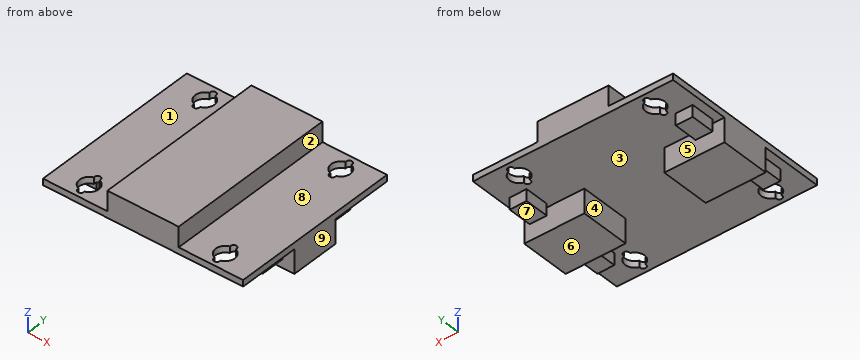
Autodesk Inventor part; units mm, degrees
ref_plane "YZ Plane" through (0, 0, 0) normal (1, 0, 0) x (0, 1, 0)
ref_plane "XZ Plane" through (0, 0, 0) normal (0, 1, 0) x (-1, 0, 0)
ref_plane "XY Plane" through (0, 0, 0) normal (0, 0, 1) x (1, 0, 0)
sketch "スケッチ1" plane through (0, 0, 0) normal (0, 0, 1) x (1, 0, 0)
  line L0 (-25, -21.59) -> (25, -21.59)
  line L1 (25, -21.59) -> (25, 21.59)
  line L2 (25, 21.59) -> (-25, 21.59)
  line L3 (-25, 21.59) -> (-25, -21.59)
  line L4 (-25, -21.59) -> (25, 21.59) construction
  line L5 (25, -21.59) -> (-25, 21.59) construction
  line L6 (-17, -17.34) -> (17, -17.34) construction
  line L7 (17, -17.34) -> (17, 17.34) construction
  line L8 (17, 17.34) -> (-17, 17.34) construction
  line L9 (-17, 17.34) -> (-17, -17.34) construction
  line L10 (-17, -17.34) -> (17, 17.34) construction
  line L11 (17, -17.34) -> (-17, 17.34) construction
  line L12 (-25, 6.2) -> (-10, 6.2)
  line L13 (-10, 6.2) -> (-10, -6.2)
  line L14 (-10, -6.2) -> (-25, -6.2)
  line L15 (-25, 0) -> (25, 0) construction
  line L16 (0, -21.59) -> (0, 21.59) construction
  line L17 (25, 6.2) -> (10, 6.2)
  line L18 (10, 6.2) -> (10, -6.2)
  line L19 (10, -6.2) -> (25, -6.2)
  line L20 (-8.89, -21.59) -> (8.89, -21.59)
  line L21 (8.89, -21.59) -> (8.89, 21.59)
  line L22 (8.89, 21.59) -> (-8.89, 21.59)
  line L23 (-8.89, 21.59) -> (-8.89, -21.59)
  line L24 (-8.89, -21.59) -> (8.89, 21.59) construction
  line L25 (8.89, -21.59) -> (-8.89, 21.59) construction
  circle A0 centre (17, 17.34) radius 2.4
  arc A1 (16.2801, 15.0505) -> (17.7199, 15.0505) centre (17, 14.84) ccw
  arc A2 (17.7199, 19.6295) -> (16.2801, 19.6295) centre (17, 19.84) ccw
  circle A3 centre (-17, 17.34) radius 2.4
  arc A4 (-16.2801, 19.6295) -> (-17.7199, 19.6295) centre (-17, 19.84) ccw
  arc A5 (-17.7199, 15.0505) -> (-16.2801, 15.0505) centre (-17, 14.84) ccw
  circle A6 centre (17, -17.34) radius 2.4
  arc A7 (16.2801, -19.6295) -> (17.7199, -19.6295) centre (17, -19.84) ccw
  arc A8 (17.7199, -15.0505) -> (16.2801, -15.0505) centre (17, -14.84) ccw
  circle A9 centre (-17, -17.34) radius 2.4
  arc A10 (-16.2801, -15.0505) -> (-17.7199, -15.0505) centre (-17, -14.84) ccw
  arc A11 (-17.7199, -19.6295) -> (-16.2801, -19.6295) centre (-17, -19.84) ccw
  line L26 (-22.86, -13.16) -> (-18.61, -13.16)
  line L27 (-18.61, -13.16) -> (-18.61, -7.16)
  line L28 (-18.61, -7.16) -> (-22.86, -7.16)
  line L29 (-22.86, -7.16) -> (-22.86, -13.16)
  line L30 (-22.86, -13.16) -> (-18.61, -7.16) construction
  line L31 (-18.61, -13.16) -> (-22.86, -7.16) construction
  line L32 (-22.86, 13.16) -> (-18.61, 13.16)
  line L33 (-18.61, 13.16) -> (-18.61, 7.16)
  line L34 (-18.61, 7.16) -> (-22.86, 7.16)
  line L35 (-22.86, 7.16) -> (-22.86, 13.16)
  line L36 (22.86, -13.16) -> (18.61, -13.16)
  line L37 (18.61, -13.16) -> (18.61, -7.16)
  line L38 (18.61, -7.16) -> (22.86, -7.16)
  line L39 (22.86, -7.16) -> (22.86, -13.16)
  line L40 (18.61, 13.16) -> (18.61, 7.16)
  line L41 (22.86, 13.16) -> (18.61, 13.16)
  line L42 (22.86, 7.16) -> (22.86, 13.16)
  line L43 (18.61, 7.16) -> (22.86, 7.16)
  point P0 (0, 0)
  point P1 (-10, 0)
  point P2 (25, 6.2)
  point P3 (25, -6.2)
  point P4 (0, 0)
  point P5 (0, 0)
  point P6 (0, 0)
  point P7 (17, 20.59)
  point P8 (17, 14.09)
  point P9 (-20.735, -10.16)
  point P10 (-22.86, -10.16)
  dimension "d0" = 50
  dimension "d1" = 43.18
  dimension "d2" = 34
  dimension "d3" = 34.68
  dimension "d8" = 15
  dimension "d9" = 12.4
  dimension "d17" = 17.78
  dimension "d18" = 43.18
  dimension "d25" = 16
  dimension "d26" = 4.8
  dimension "d27" = 6.5
  dimension "d28" = 1.5
  dimension "d29" = 1
  dimension "d30" = 8.5
  dimension "d31" = 16
  dimension "d32" = 4.25
  dimension "d33" = 6
  dimension "d34" = 10.16
  dimension "d35" = 22.86
extrude "押し出し1" add sketch "スケッチ1" along normal blind 1.6 contours L3 L14 L13 L12 L2 L23 L0 | L23 L2 L21 L0 | L3 L12 L13 L14 | L21 L2 L1 L17 L18 L19 L0 | L19 L18 L17 L1 | L29 L28 L27 L26 | L32 L33 L34 L35 | L36 L37 L38 L39 | L41 L42 L43 L40
extrude "押し出し2" add sketch "スケッチ1" against normal blind 6 contours L3 L12 L13 L14 | L19 L18 L17 L1
extrude "押し出し3" add sketch "スケッチ1" along normal blind 6.6 contours L23 L2 L21 L0
extrude "Extrusion4" add sketch "スケッチ1" against normal blind 2.9 contours L29 L28 L27 L26 | L32 L33 L34 L35 | L36 L37 L38 L39 | L41 L42 L43 L40
properties part number "SUSTAINA-STRAINGAUGE-SENSING-BOARD" material "Acetal Resin, Black"
Here's how the part is built. I have some questions about the finished solid (model axes, mm). Face numbers are marked on the shaded views. A direction names the side the tool comes from. Give positions to 0.01 mm unless a question says otherwise; leave off trailing zeros. Write each loop counter-clockwise with the first axis right and the second up, starting at its lowest first coordinate (ties: lowest second). Pieces come first, ordered by that corner, then holes.
(1) Imagine slicing it at C-C, the plane y = 9. Write out the boundary of the cut face in (x, z), and give its area (3 significant figures).
Output values:
outline: (-25, 0) - (-22.86, 0) - (-22.86, -2.9) - (-18.61, -2.9) - (-18.61, 0) - (18.61, 0) - (18.61, -2.9) - (22.86, -2.9) - (22.86, 0) - (25, 0) - (25, 1.6) - (8.89, 1.6) - (8.89, 6.6) - (-8.89, 6.6) - (-8.89, 1.6) - (-25, 1.6) - close
area: 194 mm2
(2) Thinking about a two-plate mould opening in X: for the marked faces 1, 2, 3 and 4, which applies, pulls with the +X half, pulls with the -X half, needs draft (parallel to the pull), parting line crosses it, or undercut?
Output values:
face 1: needs draft
face 2: pulls with the +X half
face 3: undercut
face 4: undercut
(3) If I drill on L1, parallel to X at y = 19.84, z = 1.1; L2, parallel to Y at x = -21.5, z = -0.5; L3, parallel to X at y = 18.5, z = 0.5, over which ranges is the centre line in solid material (lowest first)?
Output values:
L1: x = -25 to -17.75, -16.25 to 16.25, 17.75 to 25
L2: y = -13.16 to -7.16, -6.2 to 6.2, 7.16 to 13.16
L3: x = -25 to -19.1, -14.9 to 14.9, 19.1 to 25
(4) Will these pins go through, and if not, where does the flat tip stop? pin 1 (1.7 mm diameter, centred on x = -17, y = -14.84, fed in from +Z); pin 2 (2 mm diameter, centred on x = 17, y = 14.84, fed in from -Z); pin 3 (0.9 mm diameter, centred on x = 17, y = -19.84, fed in from -Z); pin 4 (1.4 mm diameter, centred on x = 21, z = -1, fed in from -Y).
Output values:
pin 1: stops at z = 1.6
pin 2: stops at z = 0
pin 3: passes through
pin 4: stops at y = -13.16
(5) On a 3-axis mill with a long thin cutter (end or side, diameter ignored), from which of +Z, -Z, +X, -X, +Y, -Y can I reach the whole of each face in a straight line? I mean the marked faces 5, 6, 7, 8 and 9. Say none if no direction works.
Output values:
face 5: -Z, +X, -X
face 6: -Z, +X, -X, +Y, -Y
face 7: -Z, +X, -X, +Y
face 8: +Z, +X, +Y, -Y
face 9: +Z, -Z, +X, +Y, -Y
(6) Imagine slicing it at B-B, the plane x = -17. Write out the boundary of the cut face in (y, z).
Output values:
outline: (-21.59, 0) - (-20.59, 0) - (-20.59, 1.6) - (-21.59, 1.6) - close; (-14.09, 0) - (-6.2, 0) - (-6.2, -6) - (6.2, -6) - (6.2, 0) - (14.09, 0) - (14.09, 1.6) - (-14.09, 1.6) - close; (20.59, 0) - (21.59, 0) - (21.59, 1.6) - (20.59, 1.6) - close
(7) Imagine slicing it at A-A, the plane z = -1.5. Write out the boundary of the cut face in (x, y).
Output values:
outline: (-25, -6.2) - (-10, -6.2) - (-10, 6.2) - (-25, 6.2) - close; (-22.86, -13.16) - (-18.61, -13.16) - (-18.61, -7.16) - (-22.86, -7.16) - close; (-22.86, 7.16) - (-18.61, 7.16) - (-18.61, 13.16) - (-22.86, 13.16) - close; (10, -6.2) - (25, -6.2) - (25, 6.2) - (10, 6.2) - close; (18.61, -13.16) - (22.86, -13.16) - (22.86, -7.16) - (18.61, -7.16) - close; (18.61, 7.16) - (22.86, 7.16) - (22.86, 13.16) - (18.61, 13.16) - close
(8) Imagine slicing it at D-D, the plane z = -4. Write out the boundary of the cut face in (x, y).
Output values:
outline: (-25, -6.2) - (-10, -6.2) - (-10, 6.2) - (-25, 6.2) - close; (10, -6.2) - (25, -6.2) - (25, 6.2) - (10, 6.2) - close
